```python
from build123d import *

# Parameters (mm, degrees)
CROQUIS2_W                         = 44
CROQUIS2_H                         = 20
BRIDA_BASE1_DEPTH                  = 1.5
BRIDA_DE_ARISTA1_STRIP_W           = 7.4732
BRIDA_DE_ARISTA1_STRIP_H           = 1.5
BRIDA_DE_ARISTA1_STRIP_CUT_DEPTH   = 20
BRIDA_DE_ARISTA1_STRIP_2_W         = 7.4732
BRIDA_DE_ARISTA1_STRIP_2_H         = 1.5
BRIDA_DE_ARISTA1_STRIP_CUT_2_DEPTH = 20
BRIDA_DE_ARISTA1_DEPTH             = 20
BRIDA_DE_ARISTA1_BEND_DEPTH        = 20
CROQUIS13_W                        = 20
CROQUIS13_H                        = 19
CORTAR_EXTRUIR1_DEPTH              = 2
BRIDA_DE_ARISTA2_DEPTH             = 39.5268
CORTAR_EXTRUIR2_START              = -22.2366
CORTAR_EXTRUIR2_OUTLINE_W          = 3.2634
CORTAR_EXTRUIR2_OUTLINE_H          = 39
CORTAR_EXTRUIR2_OUTLINE_W_2        = 1.2634
CORTAR_EXTRUIR2_DEPTH              = 2.2366
CROQUIS38_W                        = 9
CROQUIS38_H                        = 8
CORTAR_EXTRUIR3_DEPTH              = 35
BRIDA_DE_ARISTA3_DEPTH             = 20.7634
BRIDA_DE_ARISTA6_DEPTH             = 25.7634
CROQUIS51_W                        = 6.573569946
CROQUIS51_H                        = 2.7634
CROQUIS51_H_2                      = 11
CORTAR_EXTRUIR4_DEPTH              = 2
SALIENTE_EXTRUIR1_DEPTH            = 1.5
CORTAR_EXTRUIR5_DEPTH              = 51.641612746
CORTAR_EXTRUIR5_DEPTH_BACK         = 51.641612746
CROQUIS53_W                        = 1.581515027
CROQUIS53_H                        = 11
CROQUIS53_H_2                      = 2.7634
BRIDA_DE_ARISTA7_STRIP_W           = 7.4732
BRIDA_DE_ARISTA7_STRIP_H           = 1.5
BRIDA_DE_ARISTA7_STRIP_CUT_DEPTH   = 16
BRIDA_DE_ARISTA7_RELIEF_W          = 8.2232
BRIDA_DE_ARISTA7_RELIEF_H          = 0.75
BRIDA_DE_ARISTA7_RELIEF_CUT_DEPTH  = 1.5
BRIDA_DE_ARISTA7_DEPTH             = 16


# Read off the part's stored shape, not the designer's step: Cortar-Extruir2
# Sheet-metal steps are written as plain solids
with BuildPart() as part:
    # Croquis2 → Brida base1 (new body)
    with BuildSketch(Plane(origin=(0, 0, 0), x_dir=(1, 0, 0), z_dir=(0, 1, 0))):
        Rectangle(CROQUIS2_W, CROQUIS2_H)
    extrude(amount=-BRIDA_BASE1_DEPTH)

    # Brida de arista1 strip (across the edge) → Brida de arista1 strip cut (cut)
    with BuildSketch(Plane(origin=(-22, -1.5, 10), x_dir=(1, 0, 0), z_dir=(0, 0, -1))):
        with Locations((-1.5, -0.75)):
            Rectangle(BRIDA_DE_ARISTA1_STRIP_W, BRIDA_DE_ARISTA1_STRIP_H)
    extrude(amount=BRIDA_DE_ARISTA1_STRIP_CUT_DEPTH, mode=Mode.SUBTRACT)

    # Brida de arista1 strip 2 (across the edge) → Brida de arista1 strip cut 2 (cut)
    with BuildSketch(Plane(origin=(22, -1.5, -10), x_dir=(-1, 0, 0), z_dir=(0, 0, 1))):
        with Locations((-1.5, -0.75)):
            Rectangle(BRIDA_DE_ARISTA1_STRIP_2_W, BRIDA_DE_ARISTA1_STRIP_2_H)
    extrude(amount=BRIDA_DE_ARISTA1_STRIP_CUT_2_DEPTH, mode=Mode.SUBTRACT)

    # Brida de arista1 section (across the edge) → Brida de arista1 (add)
    with BuildSketch(Plane(origin=(-22, -1.5, 10), x_dir=(1, 0, 0), z_dir=(0, 0, -1))):
        with BuildLine():
            Line((0, 0.7366), (0, 27))
            Line((0, 27), (1.5, 27))
            Line((1.5, 27), (1.5, 0.7366))
            ThreePointArc((1.5, 0.7366), (1.715745145, 0.215745145), (2.2366, 0))
            Line((2.2366, 0), (2.2366, -1.5))
            ThreePointArc((2.2366, -1.5), (0.655084973, -0.844915027), (0, 0.7366))
        make_face()
    extrude(amount=BRIDA_DE_ARISTA1_DEPTH)

    # Brida de arista1 section 2 (across the edge) → Brida de arista1 bend (add)
    with BuildSketch(Plane(origin=(22, -1.5, -10), x_dir=(-1, 0, 0), z_dir=(0, 0, 1))):
        with BuildLine():
            Line((0, 0.7366), (0, 27))
            Line((0, 27), (1.5, 27))
            Line((1.5, 27), (1.5, 0.7366))
            ThreePointArc((1.5, 0.7366), (1.715745145, 0.215745145), (2.2366, 0))
            Line((2.2366, 0), (2.2366, -1.5))
            ThreePointArc((2.2366, -1.5), (0.655084973, -0.844915027), (0, 0.7366))
        make_face()
    extrude(amount=BRIDA_DE_ARISTA1_BEND_DEPTH)

    # Croquis13 → Cortar-Extruir1 (cut)
    with BuildSketch(Plane.ZY.offset(22)):
        with Locations((0, -19)):
            Rectangle(CROQUIS13_W, CROQUIS13_H)
    extrude(amount=-CORTAR_EXTRUIR1_DEPTH, mode=Mode.SUBTRACT)

    # Brida de arista2 section (across the edge) → Brida de arista2 (add)
    with BuildSketch(Plane(origin=(-19.7634, 0, 10.7366), x_dir=(0, 0, -1), z_dir=(1, 0, 0))):
        with BuildLine():
            Line((-1.5, 0.7366), (-1.5, 34.5))
            Line((-1.5, 34.5), (0, 34.5))
            Line((0, 34.5), (0, 0.7366))
            ThreePointArc((0, 0.7366), (0.215745145, 0.215745145), (0.7366, 0))
            Line((0.7366, 0), (0.7366, -1.5))
            ThreePointArc((0.7366, -1.5), (-0.844915027, -0.844915027), (-1.5, 0.7366))
        make_face()
    extrude(amount=BRIDA_DE_ARISTA2_DEPTH)

    # Cortar-Extruir2 outline → Cortar-Extruir2 (cut)
    with BuildSketch(Plane(origin=(0, 0, -10), x_dir=(-1, 0, 0), z_dir=(0, 0, -1)).offset(CORTAR_EXTRUIR2_START)):
        with Locations((18.1317, 16.5)):
            Rectangle(CORTAR_EXTRUIR2_OUTLINE_W, CORTAR_EXTRUIR2_OUTLINE_H)
        with Locations((-19.1317, 16.5)):
            Rectangle(CORTAR_EXTRUIR2_OUTLINE_W_2, CORTAR_EXTRUIR2_OUTLINE_H)
    extrude(amount=CORTAR_EXTRUIR2_DEPTH, mode=Mode.SUBTRACT)

    # Croquis38 → Cortar-Extruir3 (cut)
    with BuildSketch(Plane(origin=(0, 0, 10.7366), x_dir=(-1, 0, 0), z_dir=(0, 0, -1))):
        with Locations((12, 30.5)):
            Rectangle(CROQUIS38_W, CROQUIS38_H)
        Polygon((-1.5, 34.5), (-10.5, 34.5), (-18.5, 34.5), (-18.5, 21.5), (-10.5, 21.5), (-10.5, 29.5), (-1.5, 29.5), align=None)
    extrude(amount=-CORTAR_EXTRUIR3_DEPTH, mode=Mode.SUBTRACT)

    # Brida de arista3 section (across the edge) → Brida de arista3 (add)
    with BuildSketch(Plane(origin=(19.2366, 0.7366, 12.2366), x_dir=(-1, 0, 0), z_dir=(0, 1, 0))):
        with BuildLine():
            Line((-1.5, 0.7366), (-1.5, 6.5))
            Line((-1.5, 6.5), (0, 6.5))
            Line((0, 6.5), (0, 0.7366))
            ThreePointArc((0, 0.7366), (0.215745145, 0.215745145), (0.7366, 0))
            Line((0.7366, 0), (0.7366, -1.5))
            ThreePointArc((0.7366, -1.5), (-0.844915027, -0.844915027), (-1.5, 0.7366))
        make_face()
    extrude(amount=BRIDA_DE_ARISTA3_DEPTH)

    # Brida de arista6 section (across the edge) → Brida de arista6 (add)
    with BuildSketch(Plane(origin=(-16.80510971, 0.7366, 10.7366), x_dir=(0.7071067811865438, 0, -0.7071067811865512), z_dir=(0, 1, 0))):
        with BuildLine():
            Line((-1.5, 0.30510971), (-1.5, 6.878679656))
            Line((-1.5, 6.878679656), (0, 6.878679656))
            Line((0, 6.878679656), (0, 0.30510971))
            ThreePointArc((0, 0.30510971), (0.056070336, 0.023225094), (0.215745145, -0.215745145))
            Line((0.215745145, -0.215745145), (-0.844915027, -1.276405317))
            ThreePointArc((-0.844915027, -1.276405317), (-1.329748962, -0.550800055), (-1.5, 0.30510971))
        make_face()
    extrude(amount=BRIDA_DE_ARISTA6_DEPTH)

    # Croquis51 → Cortar-Extruir4 (cut)
    with BuildSketch(Plane(origin=(-13.770854855, 0, 13.770854855), x_dir=(-0.7071067811865513, 0, -0.7071067811865438), z_dir=(0.7071067811865438, 0, -0.7071067811865513))):
        with Locations((7.882979051, 2.1183)):
            Rectangle(CROQUIS51_W, CROQUIS51_H)
        with Locations((7.882979051, 21)):
            Rectangle(CROQUIS51_W, CROQUIS51_H_2)
    extrude(amount=-CORTAR_EXTRUIR4_DEPTH, mode=Mode.SUBTRACT)

    # Croquis52 → Saliente-Extruir1 (add)
    with BuildSketch(Plane(origin=(-13.770854855, 0, 13.770854855), x_dir=(-0.7071067811865513, 0, -0.7071067811865438), z_dir=(0.7071067811865438, 0, -0.7071067811865513))):
        Polygon((11.169764024, 15.5), (16.483472523, 20.813708499), (22.483472523, 14.813708499), (11.169764024, 3.5), align=None)
    extrude(amount=-SALIENTE_EXTRUIR1_DEPTH)

    # Croquis53 → Cortar-Extruir5 (cut, two sides: drawn at the far end of the back side and taken through both)
    with BuildSketch(Plane(origin=(0, 0, 10.7366), x_dir=(-1, 0, 0), z_dir=(0, 0, -1)).offset(-CORTAR_EXTRUIR5_DEPTH_BACK)):
        with Locations((17.290757514, 21)):
            Rectangle(CROQUIS53_W, CROQUIS53_H)
        with Locations((17.290757514, 2.1183)):
            Rectangle(CROQUIS53_W, CROQUIS53_H_2)
    extrude(amount=CORTAR_EXTRUIR5_DEPTH + CORTAR_EXTRUIR5_DEPTH_BACK, mode=Mode.SUBTRACT)

    # Brida de arista7 strip (across the edge) → Brida de arista7 strip cut (cut)
    with BuildSketch(Plane(origin=(-30.729730913, 14.813708499, -1.066700859), x_dir=(0.5000000000000012, 0.7071067811865457, 0.5000000000000013), z_dir=(0.5000000000000016, -0.7071067811865495, 0.49999999999999595))):
        with Locations((-1.5, -0.75)):
            Rectangle(BRIDA_DE_ARISTA7_STRIP_W, BRIDA_DE_ARISTA7_STRIP_H)
    extrude(amount=BRIDA_DE_ARISTA7_STRIP_CUT_DEPTH, mode=Mode.SUBTRACT)

    # Brida de arista7 relief (on the sheet) → Brida de arista7 relief cut (cut)
    with BuildSketch(Plane(origin=(-29.611430913, 16.395223526, 0.051599141), x_dir=(0.4999999999999988, 0.7071067811865457, 0.5000000000000038), z_dir=(-0.7071067811865475, -5.355429995107666e-15, 0.7071067811865478))):
        with Locations((-3.3616, -16.375)):
            Rectangle(BRIDA_DE_ARISTA7_RELIEF_W, BRIDA_DE_ARISTA7_RELIEF_H)
    extrude(amount=-BRIDA_DE_ARISTA7_RELIEF_CUT_DEPTH, mode=Mode.SUBTRACT)

    # Brida de arista7 section (across the edge) → Brida de arista7 (add)
    with BuildSketch(Plane(origin=(-30.729730913, 14.813708499, -1.066700859), x_dir=(0.5000000000000012, 0.7071067811865457, 0.5000000000000013), z_dir=(0.5000000000000016, -0.7071067811865495, 0.49999999999999595))):
        with BuildLine():
            Line((0, 0.7366), (0, 7.5))
            Line((0, 7.5), (1.5, 7.5))
            Line((1.5, 7.5), (1.5, 0.7366))
            ThreePointArc((1.5, 0.7366), (1.715745145, 0.215745145), (2.2366, 0))
            Line((2.2366, 0), (2.2366, -1.5))
            ThreePointArc((2.2366, -1.5), (0.655084973, -0.844915027), (0, 0.7366))
        make_face()
    extrude(amount=BRIDA_DE_ARISTA7_DEPTH)


solid = part.part
```
The listing builds one solid part. Answer for the finished solid, in the listing's coordinates (mm). A direction names the side the tool comes from. Coordinates: 2 decimals unless noted, no trailing zeros. Loops run counter-clockwise (first coordinate to the right, second up) from the corner with the lowest first, then second, coordinate; pieces in that order, holes last. Notation, with made-up numbers: (-18, -15) - (35, -15) arc R27 ccw to (35, 13) - close; hole circle Ø3 at (-31.75, 10.25). An arc over 180 degrees is marked (long way). Use a Markdown table: item, result. Add a question column.
1) The part is cut by section A-A, the plane y = -5.5. Give the vertices of the cut face in (x, z).
2) For faces 5 (the flat face through (6, -1, -10)), 6 (the flat face through (19.237, 11, 16)), 7 (the flat face through (18.5, 0, 11)), 8 (the flat face through (6, 29.5, 11)), 9 (the cylindrical face through (-17.345, 9.416, 12.071)), determine the directions among +Z, -Z, +X, -X, +Y, -Y from which every point of the face is accessible in a straight line to the end or side of a thin tool.
3) The mould has two halves that part along Y. Classify faces 1 (the flat face through (-24.47, 4.1, 9.52)), 2 (the flat face through (-31.128, 15.605, 0.451)), 3 (the flat face through (20, 11, 18.737)), 4 (the flat face through (-21, -9.5, 0)): released by +Y, released by -Y, zero draft, split by the parting line, or undercut.
4) Find the intervals of material crossed by line 1 (Y direction, x = -5, z = 5.25); line 2 (Z direction, x = -5, y = 12); line 3 (X direction, y = 7, z = 13.25), in increasing order.
5) The part is cut by section D-D, the plane y = -14. Give the vertices of the cut face in (x, z).
6) The part is cut by section B-B, the plane z = -7. Give the vertices of the cut face in (x, y).
7) Given pin 1 (16 mm diameter, centred on x = 7, z = 4, fed in from +Y); pin 2 (0.7 mm diameter, centred on y = 1.5, z = 11, fed in from -X); pin 3 (6.5 mm diameter, centred on y = 7.5, z = 17, fed in from -X), each flat-ended and moving along its own axis, determine where each tip first touches the part or whether it passes through.
8) The part is cut by section C-C, the plane x = -6.5. Give the vertices of the cut face in (y, z).
Here are the results:
| question | item | result |
|---|---|---|
| 1 | outline | (-22, -10) - (-20.5, -10) - (-20.5, 10) - (-22, 10) - close; (20.5, -10) - (22, -10) - (22, 10) - (20.5, 10) - close |
| 2 | face 5 | -Z, +X, -X, +Y, -Y |
| 2 | face 6 | +Z, -X, +Y, -Y |
| 2 | face 7 | +Z, +X, -Y |
| 2 | face 8 | +Z, -Z, +X, +Y |
| 2 | face 9 | +Z, +Y, -Y |
| 3 | face 1 | undercut |
| 3 | face 2 | released by +Y |
| 3 | face 3 | zero draft |
| 3 | face 4 | released by -Y |
| 4 | line 1 | y = -1.5 to 0 |
| 4 | line 2 | z = 10.74 to 12.24 |
| 4 | line 3 | x = 19.24 to 20.74 |
| 5 | outline | (20.5, -10) - (22, -10) - (22, 10) - (20.5, 10) - close |
| 6 | outline | (-22, -9.5) - (-20.5, -9.5) - (-20.5, -2.24) arc R0.74 cw to (-19.76, -1.5) - (19.76, -1.5) arc R0.74 cw to (20.5, -2.24) - (20.5, -28.5) - (22, -28.5) - (22, -2.24) arc R2.24 ccw to (19.76, 0) - (-19.76, 0) arc R2.24 ccw to (-22, -2.24) - close |
| 7 | pin 1 | stops at y = 29.5 |
| 7 | pin 2 | stops at x = -16.5 |
| 7 | pin 3 | stops at x = 19.24 |
| 8 | outline | (-1.5, -10) - (0, -10) - (0, 10) arc R0.74 cw to (0.74, 10.74) - (34.5, 10.74) - (34.5, 12.24) - (0.74, 12.24) arc R2.24 ccw to (-1.5, 10) - close |
